Autodesk Inventor part; units mm, degrees
ref_plane "YZ Plane" through (0, 0, 0) normal (1, 0, 0) x (0, 1, 0)
ref_plane "XZ Plane" through (0, 0, 0) normal (0, 1, 0) x (-1, 0, 0)
ref_plane "XY Plane" through (0, 0, 0) normal (0, 0, 1) x (1, 0, 0)
sketch "Sketch1" plane through (0, 0, 0) normal (0, 1, 0) x (-1, 0, 0)
  line L0 (-16.5491, -16.3275) -> (11.4509, -16.3275)
  line L1 (11.4509, 11.6725) -> (-16.5491, 11.6725)
  line L2 (-21.5491, 11.6725) -> (11.4509, 11.6725) construction
  line L3 (-16.5491, 6.6725) -> (-16.5491, -11.3275)
  line L4 (11.4509, 8.6725) -> (11.4509, -11.3275)
  line L5 (11.4509, -7.3275) -> (11.4509, -2.3275)
  line L6 (6.4509, -2.3275) -> (6.4509, -7.3275)
  line L7 (6.4509, -7.3275) -> (11.4509, -7.3275)
  line L8 (11.4509, 2.6725) -> (11.4509, -2.3275)
  line L9 (6.4509, -0.3275) -> (6.4509, 2.6725)
  line L10 (6.4509, 2.6725) -> (11.4509, 2.6725)
  line L11 (11.4509, -7.3275) -> (11.4509, -2.3275)
  line L12 (11.4509, -2.3275) -> (11.4509, 2.6725)
  line L13 (11.4509, 2.6725) -> (11.4509, -2.3275)
  line L14 (11.4509, -2.3275) -> (11.4509, -7.3275)
  line L15 (11.4509, -11.3275) -> (11.4509, -16.3275)
  line L16 (11.4509, 8.6725) -> (11.4509, 11.6725)
  line L17 (-2.5491, -16.3275) -> (-2.5491, 11.6725)
  circle A0 centre (-14.0491, 0.1725) radius 1
  line L18 (-11.5491, 2.6725) -> (-16.5491, 2.6725)
  line L19 (-16.5491, 2.6725) -> (-16.5491, -2.3275)
  line L20 (-16.5491, -2.3275) -> (-16.5491, 2.6725)
  line L21 (-16.5491, 2.6725) -> (-16.5491, -2.3275)
  line L22 (-11.5491, -0.3275) -> (-11.5491, 2.6725)
  circle A1 centre (-14.0491, -4.8275) radius 1.1
  line L23 (-16.5491, -7.3275) -> (-16.5491, -2.3275)
  line L24 (-16.5491, -7.3275) -> (-16.5491, -2.3275)
  line L25 (-16.5491, -2.3275) -> (-16.5491, -7.3275)
  line L26 (-11.5491, -2.3275) -> (-11.5491, -7.3275)
  line L27 (-11.5491, -7.3275) -> (-16.5491, -7.3275)
  line L28 (-16.5491, -11.3275) -> (-16.5491, -16.3275)
  line L29 (-16.5491, 8.6725) -> (-16.5491, -11.3275)
  line L30 (-16.5491, 11.6725) -> (-16.5491, -16.3275)
  line L31 (8.9509, -4.8275) -> (11.4509, -4.8275)
  line L32 (8.9509, 0.1725) -> (11.4509, 0.1725)
  circle A2 centre (8.9509, -4.8275) radius 1
  circle A3 centre (8.9509, 0.1725) radius 1.1
  point P0 (0, 0)
  point P1 (8.9509, -7.3275)
  point P2 (8.9509, 2.6725)
  point P3 (-14.0491, 2.6725)
  point P4 (-14.0491, -7.3275)
  point P5 (11.4509, 2.6725)
  point P6 (-16.5491, 2.6725)
  point P7 (11.4509, -7.3275)
  dimension "d0" = 5
  dimension "d1" = 2.5
  dimension "d2" = 2.5
  dimension "d3" = 2
  dimension "d4" = 2.2
  dimension "d5" = 2.2
  dimension "d6" = 28
  dimension "d7" = 28
  dimension "d14" = 28
extrude "Extrusion1" add sketch "Sketch1" along normal blind 5
extrude "Extrusion2" add sketch "Sketch1" along normal blind 7 contours A2 | A0
extrude "Extrusion3" add sketch "Sketch1" along normal blind 2.8 contours A3 | A1
sketch "Sketch2" plane through (0, 5, 0) normal (0, 1, 0) x (1, 0, 0)
  line L0 (-11.4509, -11.6725) -> (16.5491, -11.6725)
  line L1 (2.5491, -11.6725) -> (14.0491, -11.6725)
  line L2 (14.0491, -11.6725) -> (14.0491, -7.1725)
  line L3 (14.0491, -7.1725) -> (-8.9509, -7.1725)
  line L4 (-8.9509, -7.1725) -> (-8.9509, -11.6725)
  line L5 (2.5491, -11.6725) -> (3.2991, -11.6725)
  line L6 (3.2991, -11.6725) -> (1.7991, -11.6725)
  line L7 (1.7991, -11.6725) -> (1.7991, -7.1725)
  line L8 (1.7991, -7.1725) -> (3.2991, -7.1725)
  line L9 (3.2991, -7.1725) -> (3.2991, -11.6725)
  line L10 (3.2991, -11.6725) -> (1.7991, -11.6725)
  line L11 (-11.4509, 16.3275) -> (-11.4509, -11.6725)
  line L12 (-8.9509, -9.4225) -> (-11.4509, -9.4225)
  line L13 (-11.4509, -9.4225) -> (-11.4509, -8.4225)
  line L14 (-11.4509, -8.4225) -> (-8.9509, -8.4225)
  line L15 (-8.9509, -8.4225) -> (-8.9509, -9.4225)
  line L16 (14.0491, -9.4225) -> (14.0491, -8.4225)
  line L17 (14.0491, -8.4225) -> (16.5491, -8.4225)
  line L18 (16.5491, -8.4225) -> (16.5491, -9.4225)
  line L19 (16.5491, -9.4225) -> (14.0491, -9.4225)
  point P0 (0, 0)
  dimension "d15" = 11.5
  dimension "d16" = 4.5
  dimension "d17" = 23
  dimension "d18" = 0.75
  dimension "d19" = 1.5
  dimension "d20" = 1
extrude "Extrusion4" cut sketch "Sketch2" against normal blind 0.1 contours L4 L3 L7 L0 | L11 L14 L4 L12 | L9 L3 L2 L0 | L2 L17 L18 L19
properties part number "TracciaSotto"
The listing builds one solid part. Answer for the finished solid, in the listing's coordinates (mm). A direction names the side the tool comes from. Round coordinates to 2 decimals unless told otherwise and drop trailing zeros. Loops run counter-clockwise (first coordinate to the right, second up) from the corner with the lowest first, then second, coordinate; pieces in that order, holes last.
1) A cutting plane is placed at A-A on x = -4.5. Determine the outline of the cut face in (y, z).
Outcome:
outline: (0, -16.33) - (5, -16.33) - (5, 7.17) - (4.9, 7.17) - (4.9, 11.67) - (0, 11.67) - close
2) A cutting plane is placed at C-C on y = 5.75. Determine the outline of the cut face in (x, z).
Outcome:
outline: circle Ø2 at (-8.95, -4.83); circle Ø2 at (14.05, 0.17)
3) Consider line 1 (Z direction, x = 14.5, y = 4.75); line 2 (Y direction, x = -1.25, z = -9); line 3 (Y direction, x = 8.5, z = 10). Determine where each line is inside the solid, lowest interval first.
Outcome:
line 1: z = -16.33 to -5.83, -3.82 to 11.67
line 2: y = 0 to 5
line 3: y = 0 to 4.9
4) For faces 4 (the face through (15, 5, 11)), 5 (the face through (-9, 2.8, 0)), 6 (the face through (-9, 7, -5)), determine the directions among +Z, -Z, +X, -X, +Y, -Y from which every point of the face is accessible in a straight line to the end or side of a thin tool.
Outcome:
face 4: +Z, +X, -X, +Y
face 5: +Y
face 6: +Z, -Z, +X, -X, +Y
5) Given P1, Ø1.1, axis at x = 14, z = -5, coming from the +Y side; P2, Ø3, axis at x = 14.05, z = -4.83, coming from the +Y side, each flat-ended and moving along its own axis, determine where each tip first touches the part or whether it passes through.
Outcome:
P1: stops at y = 2.8
P2: stops at y = 5
6) A cutting plane is placed at B-B on z = -1.5. Determine the outline of the cut face in (x, y), plus the area to 3 significant figures.
Outcome:
outline: (-11.45, 0) - (16.55, 0) - (16.55, 5) - (-11.45, 5) - close
area: 140 mm2
7) For a pull along X with two mould halves and no side action, classify faces 1 (the face through (15.05, 5.99, 0.13)), 2 (the face through (14, 2.8, -5)), 3 (the face through (-10, 5, 11)) as released by +X, released by -X, zero draft, split by the parting line, or undercut.
Outcome:
face 1: split by the parting line
face 2: undercut
face 3: zero draft
